```python
from build123d import *

# Parameters (mm, degrees)
SKETCH_W     = 47
SKETCH_H     = 8
PAD_DEPTH    = 8
SKETCH001_W  = 12
SKETCH001_H  = 8
PAD001_DEPTH = 27
SKETCH002_R  = 1.5
POCKET_DEPTH = 7
CHAMFER_SIZE = 5


with BuildPart() as part:
    # Sketch → Pad (new body)
    with BuildSketch(Plane.XY):
        with Locations((23.5, 4)):
            Rectangle(SKETCH_W, SKETCH_H)
    extrude(amount=PAD_DEPTH)

    # Sketch001 (on Face8 of Pad) → Pad001 (join)
    with BuildSketch(Plane.XY.offset(8)):
        with Locations((23.5, 4)):
            Rectangle(SKETCH001_W, SKETCH001_H)
    extrude(amount=PAD001_DEPTH)

    # Sketch002 (on Face4 of Pad001) → Pocket (cut)
    with BuildSketch(Plane(origin=(0, 0, 0), x_dir=(1, 0, 0), z_dir=(0, 0, -1))):
        with Locations((36, -4)):
            Circle(SKETCH002_R)
        with Locations((11, -4)):
            Circle(SKETCH002_R)
    extrude(amount=-POCKET_DEPTH, mode=Mode.SUBTRACT)

    # Chamfer
    chamfer_edges = [part.edges().sort_by_distance(p)[0] for p in [
        (17.5, 4, 8),
        (29.5, 4, 8),
    ]]
    chamfer(chamfer_edges, length=CHAMFER_SIZE)


solid = part.part
```
Here's how the part is built. I have some questions about the finished solid (model axes, mm). A direction names the side the tool comes from. Give positions to 0.01 mm unless a question says otherwise; leave off trailing zeros. Write each loop counter-clockwise with the first axis right and the second up, starting at its lowest first coordinate (ties: lowest second). Pieces come first, ordered by that corner, then holes. Notation, with made-up numbers: (72, 38) -> (89, 38) arc R25 ccw to (89, 50) -> close; hole circle Ø9 at (19, 79). An arc over 180 degrees is marked (long way). Use one line per item in the form item = value.
1) Suppose I cut it at D-D (z = 9). Please give me the cut outline in (x, y), and give its area (3 significant figures).
Verdict:
outline = (13.5, 0) -> (33.5, 0) -> (33.5, 8) -> (13.5, 8) -> close
area = 160 mm2
2) Suppose I cut it at B-B (y = 4). Please give me the cut outline in (x, z), and give its area (3 significant figures).
Verdict:
outline = (0, 0) -> (9.5, 0) -> (9.5, 7) -> (12.5, 7) -> (12.5, 0) -> (34.5, 0) -> (34.5, 7) -> (37.5, 7) -> (37.5, 0) -> (47, 0) -> (47, 8) -> (34.5, 8) -> (29.5, 13) -> (29.5, 35) -> (17.5, 35) -> (17.5, 13) -> (12.5, 8) -> (0, 8) -> close
area = 683 mm2
3) Suppose I cut it at A-A (z = 3.5). Please give me the cut outline in (x, y).
Verdict:
outline = (0, 0) -> (47, 0) -> (47, 8) -> (0, 8) -> close; hole circle Ø3 at (11, 4); hole circle Ø3 at (36, 4)
4) I'm going to push flat-ended pins straight in: pin 1 (2.5 mm diameter, centred on y = 4.5, z = 24.5, fed in from -X); pin 2 (6 mm diameter, centred on x = 34, z = 18.5, fed in from -Y); pin 3 (2.5 mm diameter, centred on x = 36, y = 4, fed in from -Z); pin 4 (4 mm diameter, centred on x = 9, y = 4.5, fed in from +Z). Where does each tip first touch, or does it pass through?
Verdict:
pin_1 = 17.5
pin_2 = through
pin_3 = 7
pin_4 = 8
5) We'd pull the mould along Y, two halves only. Please class faces 5 (the face through (23, 0, 13)), 6 (the face through (11, 4, 7)), 7 (the face through (17.5, 4, 24)), 8 (the face through (23, 8, 13)): +Y half, -Y half, draft (parallel to the pull), parting line (faces both ways), or undercut.
Verdict:
face_5 = -Y half
face_6 = undercut
face_7 = draft
face_8 = +Y half
6) Suppose I cut it at C-C (x = 36). Please give me the cut outline in (y, z).
Verdict:
outline = (0, 0) -> (2.5, 0) -> (2.5, 7) -> (5.5, 7) -> (5.5, 0) -> (8, 0) -> (8, 8) -> (0, 8) -> close
7) On a 3-axis mill with a long thin cutter (end or side, diameter ignored), from which of +Z, -Z, +X, -X, +Y, -Y can I reach the whole of each face in a straight line? I mean faces 1 (the face through (23, 4, 0)), 2 (the face through (34.8, 4.9, 3.5)), 3 (the face through (29.5, 4, 24)), 4 (the face through (6, 4, 8)). Say none if no direction works.
Verdict:
face_1 = -Z, +X, -X, +Y, -Y
face_2 = -Z
face_3 = +Z, +X, +Y, -Y
face_4 = +Z, -X, +Y, -Y
8) If I drill on L1, parallel to X at y = 4, z = 2.25; L2, parallel to Y at x = 11, z = 3.25; L3, parallel to X at y = 4, z = 14, over which ranges is the centre line in solid material (lowest first)? Write a range as [from, to].
Verdict:
L1 = [0, 9.5], [12.5, 34.5], [37.5, 47]
L2 = [0, 2.5], [5.5, 8]
L3 = [17.5, 29.5]
